Source: CAD feature listing. Evaluate the final solid. Frame: model axes, mm. Round coordinates to 2 decimals unless told otherwise and drop trailing zeros. Order: outer loops, then holes, each group sorted by start corner. A loop starts at its lowest first (then second) coordinate and runs counter-clockwise, first axis right, second up. Notation, with made-up numbers: M -37.5,-13 L -16.5,-13 A15 cw -16.5,2 Z; hole C 46,45.25 d6. An arc over 180 degrees is marked long. Use one line per item in the form item = value. Start each with the question number.
Q1. Section C-C (z = 2.75). Return the cut outline in (x, y) (3 decimals).
Q2. Section A-A (y = -100). Return the cut outline in (x, z) (1 decimal), plus the area to 3 significant figures.
Q3. Material intervals for probe 1 along X at (y, z) = (-23, 4) (3 decimals); probe 2 along Y at (x, z) = (-96, 4.5) (3 decimals); probe 3 along Z at (x, y) = (162, 108) (1 decimal), sorted ascending.
Q4. Section D-D (y = 4). Return the cut outline in (x, z) (1 decimal), plus the area to 3 significant figures.
Q5. Section B-B (x = 27). Return the cut outline in (y, z) (1 decimal), plus the area to 3 significant figures.
Q6. Contact query for flat-ended pins moving along their axis: pin 1 (1.8 mm diameter, centred on x = -78, z = 4, fed in from +Y) (3 decimals); pin 2 (3 mm diameter, centred on y = -6, z = 4, fed in from +X); pin 3 (3 mm diameter, centred on y = -21.5, z = 3, fed in from -X); pin 4 (5 mm diameter, centred on x = 4, z = 4, fed in from +Y) (3 decimals). Output: stop coordinate, or through.
from build123d import *

# Parameters (mm, degrees)
F1_W      = 603.25
F1_H      = 234.95
F2_DEPTH  = 12.065
F3_W      = 12.065
F3_H      = 234.95
F4_DEPTH  = 6.0325
F5_W      = 12.065
F5_H      = 234.95
F6_DEPTH  = 6.0325
F7_W      = 12.065
F7_H      = 234.95
F8_DEPTH  = 6.0325
F9_W      = 12.065
F9_H      = 234.95
F10_DEPTH = 6.0325
F11_W     = 203.2
F11_H     = 12.065
F14_DEPTH = 6.0325
F12_W     = 148.59
F12_H     = 12.065
F15_DEPTH = 6.0325
F13_W     = 203.2
F13_H     = 12.065
F16_DEPTH = 6.0325
F17_W     = 12.065
F17_H     = 31.75
F18_DEPTH = 6.0325
F19_W     = 12.065
F19_H     = 31.75
F20_DEPTH = 6.0325


# Not quite as in the source:
# - a variable given as a bare number and used for a length is read in inches; the dataset says mm whatever the document's units were


with BuildPart() as f2:
    # F1 (on Top) → F2 (new body)
    with BuildSketch(Plane.XY):
        Rectangle(F1_W, F1_H)
    extrude(amount=F2_DEPTH)

    # F3 (on face) → F4 (cut)
    with BuildSketch(Plane(origin=(0, 0, 0), x_dir=(1, 0, 0), z_dir=(0, 0, -1))):
        with Locations((-295.5925, 0)):
            Rectangle(F3_W, F3_H)
    extrude(amount=-F4_DEPTH, mode=Mode.SUBTRACT)

    # F5 (on face) → F6 (cut)
    with BuildSketch(Plane(origin=(0, 0, 0), x_dir=(1, 0, 0), z_dir=(0, 0, -1))):
        with Locations((295.5925, 0)):
            Rectangle(F5_W, F5_H)
    extrude(amount=-F6_DEPTH, mode=Mode.SUBTRACT)

    # F7 (on face) → F8 (cut)
    with BuildSketch(Plane(origin=(0, 0, 0), x_dir=(1, 0, 0), z_dir=(0, 0, -1))):
        with Locations((80.3275, 0)):
            Rectangle(F7_W, F7_H)
    extrude(amount=-F8_DEPTH, mode=Mode.SUBTRACT)

    # F9 (on face) → F10 (cut)
    with BuildSketch(Plane(origin=(0, 0, 0), x_dir=(1, 0, 0), z_dir=(0, 0, -1))):
        with Locations((-80.3275, 0)):
            Rectangle(F9_W, F9_H)
    extrude(amount=-F10_DEPTH, mode=Mode.SUBTRACT)

    # F11 (on face) → F14 (cut)
    with BuildSketch(Plane(origin=(0, 0, 0), x_dir=(1, 0, 0), z_dir=(0, 0, -1))):
        with Locations((187.96, -111.4425)):
            Rectangle(F11_W, F11_H)
    extrude(amount=-F14_DEPTH, mode=Mode.SUBTRACT)

    # F12 (on face) → F15 (cut)
    with BuildSketch(Plane(origin=(0, 0, 0), x_dir=(1, 0, 0), z_dir=(0, 0, -1))):
        with Locations((0, -111.4425)):
            Rectangle(F12_W, F12_H)
    extrude(amount=-F15_DEPTH, mode=Mode.SUBTRACT)

    # F13 (on face) → F16 (cut)
    with BuildSketch(Plane(origin=(0, 0, 0), x_dir=(1, 0, 0), z_dir=(0, 0, -1))):
        with Locations((-187.96, -111.4425)):
            Rectangle(F13_W, F13_H)
    extrude(amount=-F16_DEPTH, mode=Mode.SUBTRACT)

    # F17 (on face) → F18 (join)
    with BuildSketch(Plane(origin=(0, 0, 6.0325), x_dir=(1, 0, 0), z_dir=(0, 0, -1))):
        with Locations((80.3275, 101.6)):
            Rectangle(F17_W, F17_H)
    extrude(amount=F18_DEPTH)

    # F19 (on face) → F20 (join)
    with BuildSketch(Plane(origin=(0, 0, 6.0325), x_dir=(1, 0, 0), z_dir=(0, 0, -1))):
        with Locations((-80.3275, 101.6)):
            Rectangle(F19_W, F19_H)
    extrude(amount=F20_DEPTH)


solid = f2.part
Results list:
q1.outline = M -289.56,-117.475 L 289.56,-117.475 L 289.56,105.41 L 86.36,105.41 L 86.36,-85.725 L 74.295,-85.725 L 74.295,105.41 L -74.295,105.41 L -74.295,-85.725 L -86.36,-85.725 L -86.36,105.41 L -289.56,105.41 Z
q2.outline = M -301.6,6 L -289.6,6 L -289.6,0 L 289.6,0 L 289.6,6 L 301.6,6 L 301.6,12.1 L -301.6,12.1 Z
q2.area = 7,130 mm2
q3.probe_1 = -289.56 to -86.36, -74.295 to 74.295, 86.36 to 289.56
q3.probe_2 = -117.475 to 105.41
q3.probe_3 = 6 to 12.1
q4.outline = M -301.6,6 L -289.6,6 L -289.6,0 L -86.4,0 L -86.4,6 L -74.3,6 L -74.3,0 L 74.3,0 L 74.3,6 L 86.4,6 L 86.4,0 L 289.6,0 L 289.6,6 L 301.6,6 L 301.6,12.1 L -301.6,12.1 Z
q4.area = 6,990 mm2
q5.outline = M -117.5,0 L 105.4,0 L 105.4,6 L 117.5,6 L 117.5,12.1 L -117.5,12.1 Z
q5.area = 2,760 mm2
q6.pin_1 = -85.725
q6.pin_2 = 289.56
q6.pin_3 = -289.56
q6.pin_4 = 117.475
